The model under review builds one solid part; all positions refer to its coordinate system, in mm. A direction names the side the tool comes from. Round coordinates to 2 decimals unless told otherwise and drop trailing zeros. Write each loop counter-clockwise with the first axis right and the second up, starting at its lowest first coordinate (ties: lowest second). Pieces come first, ordered by that corner, then holes. Notation, with made-up numbers: (46, 57.25) - (67, 57.25) arc R7 cw to (67, 66.25) - close; hole circle Ø8 at (-32, 42.5). An arc over 180 degrees is marked (long way). Return JSON: item names as keys, results as strings.
Autodesk Inventor part; units mm, degrees
ref_plane "YZ Plane" through (0, 0, 0) normal (1, 0, 0) x (0, 1, 0)
ref_plane "XZ Plane" through (0, 0, 0) normal (0, 1, 0) x (-1, 0, 0)
ref_plane "XY Plane" through (0, 0, 0) normal (0, 0, 1) x (1, 0, 0)
sketch "Sketch1" plane through (0, 0, 0) normal (0, 0, 1) x (1, 0, 0)
  line L0 (0, 0) -> (139.7, 0)
  line L1 (139.7, 0) -> (139.7, 117.475)
  line L2 (139.7, 117.475) -> (0, 117.475)
  line L3 (0, 117.475) -> (0, 0)
  dimension "d0" = 139.7
  dimension "d1" = 117.475
extrude "Plate3" add sketch "Sketch1" along normal blind 3.048
sketch "Sketch4" plane through (0, 0, 0) normal (0, 0, -1) x (-1, 0, 0)
  circle A0 centre (-22.86, 79.375) radius 31.242
  circle A1 centre (-6.35, 111.125) radius 2.5527
  circle A2 centre (-6.35, 47.625) radius 2.5527
  circle A3 centre (-133.35, 111.125) radius 2.5527
  circle A4 centre (-133.35, 47.625) radius 2.5527
  arc A5 (-136.4869, 13.4874) -> (-136.4869, 27.7876) centre (-136.4869, 20.6375) ccw
  line L0 (-150.7617, 27.7876) -> (-136.4869, 27.7876)
  line L1 (-136.4869, 13.4874) -> (-150.7617, 13.4874)
  arc A6 (-99.9617, 27.7876) -> (-99.9617, 13.4874) centre (-99.9617, 20.6375) ccw
  line L2 (-99.9617, 27.7876) -> (-85.6869, 27.7876)
  line L3 (-85.6869, 13.4874) -> (-99.9617, 13.4874)
  arc A7 (-85.6869, 13.4874) -> (-85.6869, 27.7876) centre (-85.6869, 20.6375) ccw
  arc A8 (-49.1617, 27.7876) -> (-49.1617, 13.4874) centre (-49.1617, 20.6375) ccw
  line L4 (-49.1617, 27.7876) -> (-34.8869, 27.7876)
  arc A9 (-34.8869, 13.4874) -> (-34.8869, 27.7876) centre (-34.8869, 20.6375) ccw
  line L5 (-34.8869, 13.4874) -> (-49.1617, 13.4874)
  arc A10 (1.6383, 27.7876) -> (1.6383, 13.4874) centre (1.6383, 20.6375) ccw
  line L6 (1.6383, 27.7876) -> (15.9131, 27.7876)
  line L7 (15.9131, 13.4874) -> (1.6383, 13.4874)
  arc A11 (15.9131, 13.4874) -> (15.9131, 27.7876) centre (15.9131, 20.6375) ccw
  circle A12 centre (-104.2924, 79.375) radius 15.5575
  circle A13 centre (-63.5762, 79.375) radius 12.095
  circle A14 centre (-22.86, 79.375) radius 31.242
  circle A15 centre (-6.35, 47.625) radius 2.5527
  circle A16 centre (-63.5762, 79.375) radius 12.095
  circle A17 centre (-104.2924, 79.375) radius 15.5575
  circle A18 centre (-133.35, 111.125) radius 2.5527
  circle A19 centre (-133.35, 47.625) radius 2.5527
  circle A20 centre (-6.35, 111.125) radius 2.5527
  circle A21 centre (-92.8243, 20.6375) radius 3.175
  circle A22 centre (-42.0243, 20.6375) radius 3.175
  point P0 (0, 0)
  dimension "d16" = 7.1501
  dimension "d17" = 7.1501
  dimension "d18" = 7.1374
  dimension "d19" = 7.1374
  dimension "d20" = 6.35
  dimension "d21" = 6.35
extrude "Cut1" cut sketch "Sketch4" against normal blind 3.048 contours A0 A13 | A13 A0 | A0 A13 | A1 | A2 | A3 | A4 | A12 | A21 | A22
equation "\"d12\" = Thickness"
equation "\"BendRadius\" = Thickness"
equation "\"BendReliefWidth\" = Thickness"
equation "\"BendReliefDepth\" = 0.5 * Thickness"
equation "\"CornerReliefSize\" = 4 * Thickness"
equation "\"MinimumRemnant\" = 2 * Thickness"
equation "\"TransitionRadius\" = BendRadius"
equation "\"JacobiRadiusSize\" = BendRadius"
equation "\"GapSize\" = Thickness"
equation "\"d2\" = BendRadius"
equation "\"d3\" = BendRadius"
equation "\"d4\" = BendRadius"
properties part number "attatching plate for toughbox"
(1) Wall thickness on line 1 (X direction, y = 20.5, z = 2.3); line 2 (Y direction, x = 133.35, z = 1) (3 decimals); line 3 (Y direction, x = 63, z = 0.45) (3 decimals): over which ranges is each line inside the solid? List them lowest first.
Filled in:
{"line 1": "x = 0 to 38.85, 45.2 to 89.65, 96 to 139.7", "line 2": "y = 0 to 45.072, 50.178 to 108.572, 113.678 to 117.475", "line 3": "y = 0 to 67.294, 91.456 to 117.475"}
(2) Clearance check with a flat-ended pin moving along its axis: pin 1 Ø1.5 at (x, z) = (89.5, 2.5) entering from -Y. State where the tip first meets the part, or that it passes through.
Filled in:
{"pin 1": "stops at y = 0"}
(3) For faces 1 (the flat face through (0, 29, 2)), 2 (the cylindrical face through (31.63, 49.39, 1.5)), list the 3-axis set-ups (+Z, -Z, +X, -X, +Y, -Y) from which the entire face can be reached by the end or side of a thin tool; tool diameter is ignored.
Filled in:
{"face 1": "+Z, -Z, -X, +Y, -Y", "face 2": "+Z, -Z"}
(4) Add section B-B (y = 105.5). Write out the cut boundary in (x, z), plus the area to 3 significant figures.
Filled in:
{"outline": "(0, 0) - (5.73, 0) - (5.73, 3.05) - (0, 3.05) - close; (39.99, 0) - (139.7, 0) - (139.7, 3.05) - (39.99, 3.05) - close", "area": "321 mm2"}
(5) Mouldability with a two-part tool opening along Y and no side actions: class faces 3 (the flat face through (0, 109, 2)), 4 (the cylindrical face through (30.714, 109.614, 1.503)), 5 (the flat face through (69, 0, 2)), 6 (the cylindrical face through (135.9, 111.2, 1.5)) as released by +Y, released by -Y, zero draft, split by the parting line, or undercut.
Filled in:
{"face 3": "zero draft", "face 4": "undercut", "face 5": "released by -Y", "face 6": "undercut"}
(6) Add section D-D (z = 0.6). Give the number of separate pieces and of enclosed holes in the cut face, plus the area to 3 significant figures.
Filled in:
{"separate pieces": "1", "enclosed holes": "7", "area": "12,200 mm2"}
(7) Add section C-C (x = 6.35). Write out the cut boundary in (y, z) (3 decimals), plus the area to 3 significant figures.
Filled in:
{"outline": "(0, 0) - (45.072, 0) - (45.072, 3.048) - (0, 3.048) - close; (50.178, 0) - (52.852, 0) - (52.852, 3.048) - (50.178, 3.048) - close; (105.898, 0) - (108.572, 0) - (108.572, 3.048) - (105.898, 3.048) - close; (113.678, 0) - (117.475, 0) - (117.475, 3.048) - (113.678, 3.048) - close", "area": "165 mm2"}
(8) Add section A-A (x = 133.35). Write out the cut boundary in (y, z) (3 decimals).
Filled in:
{"outline": "(0, 0) - (45.072, 0) - (45.072, 3.048) - (0, 3.048) - close; (50.178, 0) - (108.572, 0) - (108.572, 3.048) - (50.178, 3.048) - close; (113.678, 0) - (117.475, 0) - (117.475, 3.048) - (113.678, 3.048) - close"}
